Autodesk Inventor part; units mm, degrees
ref_plane "Work Plane1" through (-21.4473, 101.6, -11.1519) normal (-1, 0, 0) x (0, -1, 0)
ref_plane "Work Plane2" through (24.2727, 101.6, -11.1519) normal (-1, 0, 0) x (0, -1, 0)
ref_plane "YZ Plane" through (0, 0, 0) normal (1, 0, 0) x (0, 1, 0)
sketch "Sketch1" plane through (0, 0, 0) normal (0, 1, 0) x (-1, 0, 0)
  line L0 (-24.3078, -15.4178) -> (21.4122, -15.4178)
  line L1 (21.4122, 12.5222) -> (-24.3078, 12.5222)
  arc A0 (21.4122, -15.4178) -> (21.4122, 12.5222) centre (21.4122, -1.4478) ccw
  arc A1 (-24.3078, 12.5222) -> (-24.3078, -15.4178) centre (-24.3078, -1.4478) ccw
  point P0 (0, 0)
  dimension "d2" = 27.94
  dimension "d3" = 45.72
extrude "Extrusion1" add sketch "Sketch1" along normal blind 101.6
sketch "Sketch2" plane through (0, 101.6, 0) normal (0, 1, 0) x (1, 0, 0)
  line L0 (24.2727, 11.1519) -> (-21.4473, 11.1519)
  line L1 (-21.4473, -9.1681) -> (24.2727, -9.1681)
  arc A0 (-21.4473, 11.1519) -> (-21.4473, -9.1681) centre (-21.4473, 0.9919) ccw
  arc A1 (24.2727, -9.1681) -> (24.2727, 11.1519) centre (24.2727, 0.9919) ccw
  arc A2 (-21.4122, 15.4178) -> (-21.4122, -12.5222) centre (-21.4122, 1.4478) ccw
  point P0 (0, 0)
  dimension "d7" = 20.32
  dimension "d8" = 45.72
extrude "Extrusion2" cut sketch "Sketch2" against normal blind 95.25
sketch "Sketch3" plane through (0, 6.35, 0) normal (0, 1, 0) x (1, 0, 0)
  arc A0 (-21.4122, 15.4178) -> (-21.4122, -12.5222) centre (-21.4122, 1.4478) ccw
  line L0 (-33.8556, -4.9022) -> (40.6958, -4.9022)
  line L1 (40.6958, -4.9022) -> (40.6958, -12.5222)
  line L2 (40.6958, -12.5222) -> (-33.8556, -12.5222)
  line L3 (-33.8556, -12.5222) -> (-33.8556, -4.9022)
  line L4 (-21.4122, -12.5222) -> (24.3078, -12.5222)
  point P0 (0, 0)
  dimension "d13" = 7.62
  dimension "d14" = 0
extrude "Extrusion3" cut sketch "Sketch3" along normal blind 95.25
fillet "Fillet1" [suppressed]
ref_plane "Work Plane1" through (-21.4473, 101.6, -11.1519) normal (-1, 0, 0) x (0, -1, 0)
ref_plane "Work Plane2" through (24.2727, 101.6, -11.1519) normal (-1, 0, 0) x (0, -1, 0)
sketch "Sketch6" plane through (24.2727, 101.6, -11.1519) normal (-1, 0, 0) x (0, -1, 0)
  line L0 (66.929, 0.4433) -> (32.131, 0.4433)
  line L1 (32.131, 0.4433) -> (32.131, 26.3545)
  line L2 (32.131, 26.3545) -> (66.929, 26.3545)
  line L3 (66.929, 26.3545) -> (66.929, 0.4433)
  line L4 (95.25, 16.0541) -> (95.25, 23.6741)
  point P0 (101.6, 11.1519)
  point P1 (95.25, 16.0541)
  dimension "d30" = 34.798
  dimension "d31" = 28.321
extrude "Extrusion6" cut sketch "Sketch6" against normal up to next
sketch "Sketch7" plane through (-21.4473, 101.6, -11.1519) normal (-1, 0, 0) x (0, -1, 0)
  line L0 (31.75, 1.1631) -> (66.04, 1.1631)
  line L1 (66.04, 1.1631) -> (66.04, 21.3162)
  line L2 (66.04, 21.3162) -> (31.75, 21.3162)
  line L3 (31.75, 21.3162) -> (31.75, 1.1631)
  line L4 (95.25, 16.0541) -> (95.25, 23.6741)
  point P0 (101.6, 11.1519)
  dimension "d35" = 34.29
  dimension "d36" = 29.21
extrude "Extrusion7" cut sketch "Sketch7" along normal blind 25.4
sketch "Sketch10" plane through (-21.4473, 101.6, -11.1519) normal (0, 0, 1) x (1, 0, 0)
  line L0 (-13.9903, -31.75) -> (1.8847, -31.75)
  line L1 (1.8847, -31.75) -> (1.8847, -66.04)
  line L2 (1.8847, -66.04) -> (-13.9903, -66.04)
  line L3 (-13.9903, -66.04) -> (-13.9903, -31.75)
  line L4 (59.7251, -101.6) -> (59.7251, 0)
  line L5 (59.7251, -32.131) -> (43.8501, -32.131)
  line L6 (43.8501, -32.131) -> (43.8501, -66.929)
  line L7 (43.8501, -66.929) -> (59.7251, -66.929)
  line L8 (59.7251, -66.929) -> (59.7251, -32.131)
  line L9 (53.9955, -32.131) -> (58.1985, -32.131)
  point P0 (21.4473, -101.6)
  point P1 (55.1473, -32.131)
  dimension "d58" = 15.875
  dimension "d59" = 34.29
  dimension "d60" = 15.875
  dimension "d61" = 34.798
  dimension "d62" = 0
extrude "Extrusion10" cut sketch "Sketch10" against normal through all both and the other way through all
fillet "Fillet6" radius 6.35 4 edges at (22.4028, 69.469, -13.2849) (22.4028, 34.671, -13.2849) (-19.5625, 69.85, -13.2849) (-19.5625, 35.56, -13.2849)
sketch "Sketch11" plane through (0, 6.35, 0) normal (0, 1, 0) x (1, 0, 0)
  arc A0 (32.5483, -4.9022) -> (24.2727, 11.1519) centre (24.2727, 0.9919) ccw
  arc A1 (24.2727, -10.5778) -> (24.2727, 12.5616) centre (24.2727, 0.9919) ccw
  arc A2 (-21.4473, 11.1519) -> (-29.7228, -4.9022) centre (-21.4473, 0.9919) ccw
  arc A3 (-21.4473, 12.5616) -> (-20.3359, -10.5243) centre (-21.4473, 0.9919) ccw
  line L0 (24.2727, 12.5616) -> (-24.2727, 12.5616)
  line L1 (-20.4393, -10.5778) -> (24.2727, 12.5616) construction
  line L2 (20.4393, -10.5778) -> (-24.2727, 12.5616) construction
  line L3 (24.2727, -10.5778) -> (-21.4473, -10.5778)
  line L4 (-24.2727, 12.5616) -> (-24.2727, 10.7512)
  line L5 (24.2727, 0.9919) -> (24.2727, 12.5616)
  point P0 (0, 0)
  point P1 (33.1455, -3.9578)
  point P2 (-30.32, -3.9578)
  dimension "d66" = 23.1394
  dimension "d67" = 23.1394
extrude "Extrusion11" cut sketch "Sketch11" along normal blind 6.35 contours L3 A3 L0 A1
properties part number "Proto-Valve Holder"
Can you work these out from the model? Positions are in its coordinate system, mm. A direction names the side the tool comes from. Round coordinates to 2 decimals unless told otherwise and drop trailing zeros. Write each loop counter-clockwise with the first axis right and the second up, starting at its lowest first coordinate (ties: lowest second). Pieces come first, ordered by that corner, then holes. Notation, with made-up numbers: (32, 60) -> (46, 60) arc R34 ccw to (46, 97) -> close; hole circle Ø6 at (10, 66.5). An arc over 180 degrees is marked (long way). Use one line per item in the form item = value. Start each with the question number.
Q1. Imagine slicing it at A-A (y = 33). Please give me the cut outline in (x, z).
Q2. I'm going to push flat-ended pins straight in: P1, Ø4.5, axis at y = 58, z = -12.5, coming from the -X side; P2, Ø10, axis at x = 3.5, z = 0, coming from the +Y side; P3, Ø1.2, axis at x = -31.5, y = 91.5, coming from the +Z side. Where does each tip first touch, or does it pass through?
Q3. Imagine slicing it at C-C (x = 14). Please give me the cut outline in (y, z), then the cut area to 3 significant figures.
Q4. If I drill on probe 1 along Z at (x, y) = (10.5, 63); probe 2 along Y at (x, z) = (-23, 11.25); probe 3 along Y at (x, z) = (26, -12.75), over which ranges is the centre line in solid material (lowest first)? Write a range as [from, to].
Q5. We'd pull the mould along X, two halves only. Please class faces 5 (the face through (37.33, 17.99, -6.51)), 6 (the face through (2, 0, -1)), 7 (the face through (-30.41, 85.04, -5.78)): +X half, -X half, draft (parallel to the pull), parting line (faces both ways), or undercut.
Q6. Which directions (+Z, -Z, +X, -X, +Y, -Y) give clear straight access to the entire face, cutting with the end or side of a thin tool? Please do faces 1 (the face through (2, 9, -12.562)), 2 (the face through (35, 69.469, -5)), 3 (the face through (34.24, 9.48, -6.87)), 4 (the face through (-21.373, 37.47, -13.394)).
Q7. Imagine slicing it at D-D (x = 26). Please give me the cut outline in (y, z).
Q8. Imagine slicing it at B-B (z = 1.75). Please give me the cut outline in (x, y), then the cut area to 3 significant figures.
Worked out:
q1.outline = (-33.86, 4.9) arc R13.97 ccw to (-21.41, -15.42) -> (24.31, -15.42) arc R13.97 ccw to (36.75, 4.9) -> (32.55, 4.9) arc R10.16 cw to (24.27, -11.15) -> (-21.45, -11.15) arc R10.16 cw to (-29.72, 4.9) -> close
q2.P1 = -19.56
q2.P2 = 6.35
q2.P3 = 4.9
q3.outline = (0, -15.42) -> (101.6, -15.42) -> (101.6, -11.15) -> (12.7, -11.15) -> (12.7, -12.56) -> (6.35, -12.56) -> (6.35, 12.52) -> (0, 12.52) -> close
q3.area = 575 mm^2
q4.probe_1 = [-15.42, -11.15]
q4.probe_2 = [0, 6.35]
q4.probe_3 = [0, 35.3], [68.84, 101.6]
q5.face_5 = +X half
q5.face_6 = draft
q5.face_7 = undercut
q6.face_1 = +Z
q6.face_2 = +Z, -Z, +X
q6.face_3 = none
q6.face_4 = +Z, -Z, -X
q7.outline = (0, -15.31) -> (35.3, -15.31) -> (35.3, -11) -> (12.7, -11) -> (12.7, -12.43) -> (6.35, -12.43) -> (6.35, 12.42) -> (0, 12.42) -> close; (68.84, -15.31) -> (101.6, -15.31) -> (101.6, -11) -> (68.84, -11) -> close
q8.outline = (-35.01, 0) -> (37.91, 0) -> (37.91, 34.67) -> (34.06, 34.67) -> (34.06, 12.7) -> (35.51, 12.7) -> (35.51, 6.35) -> (-32.69, 6.35) -> (-32.69, 12.7) -> (-31.23, 12.7) -> (-31.23, 35.56) -> (-35.01, 35.56) -> close; (-35.01, 69.85) -> (-31.23, 69.85) -> (-31.23, 101.6) -> (-35.01, 101.6) -> close; (34.06, 69.47) -> (37.91, 69.47) -> (37.91, 101.6) -> (34.06, 101.6) -> close
q8.area = 908 mm^2
